Check sheet for the drawn part. Datum: minimum x, y, z corner. Units: mm. Round coordinates to 2 decimals unless told otherwise and drop trailing zeros. Loops run counter-clockwise (first coordinate to the right, second up) from the corner with the lowest first, then second, coordinate; pieces in that order, holes last. Notation, with made-up numbers: (64, 85) -> (121, 85) arc R19 ccw to (121, 109) -> close; hole circle Ø10 at (-18, -23.75). An arc over 180 degrees is marked (long way). Return JSON: item names as keys, results as strings.
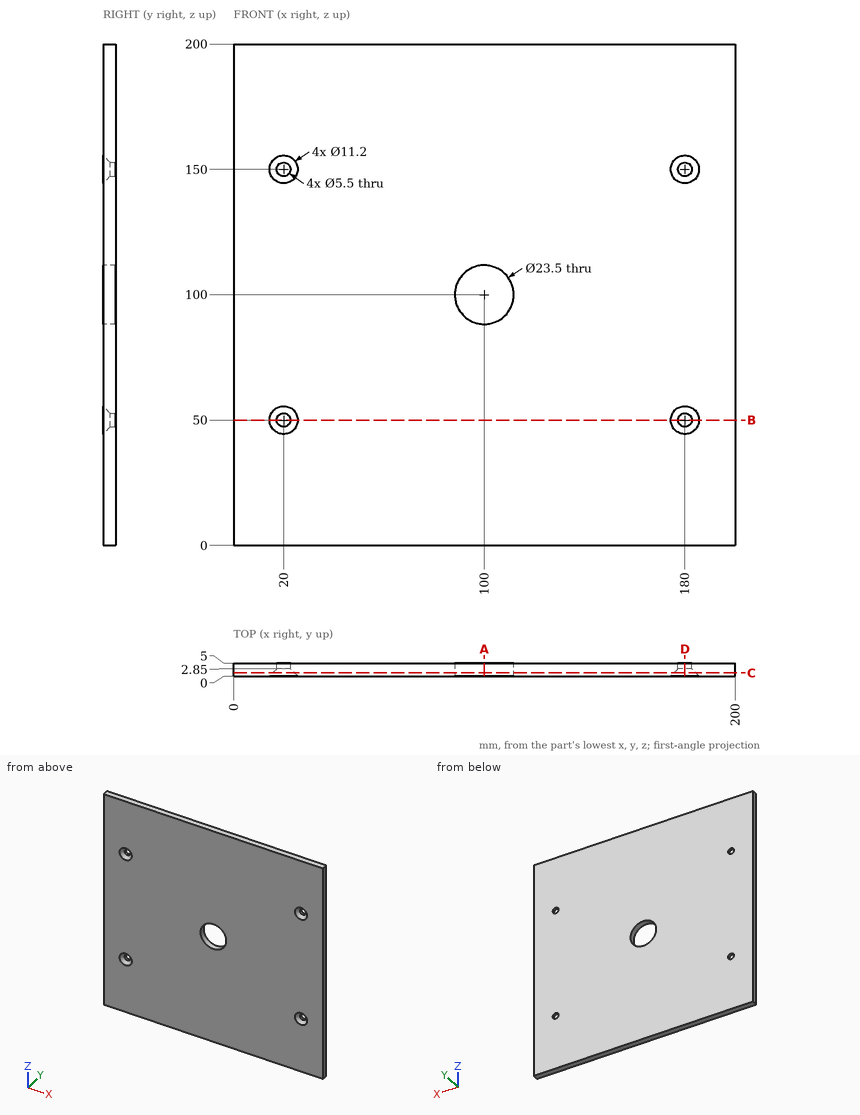
Q1. Go/stop test with flat-tipped pins: pin 1 (4.5 mm diameter, centred on x = 180, z = 150, fed in from +Y); pin 2 (10 mm diameter, centred on x = 163.5, z = 29, fed in from -Y). Record where each tip stops, or that it passes through.
Results list:
{"pin 1": "through", "pin 2": "y = 0"}
Q2. Section check A-A (x = 100). Record the boundary of the cut face in (y, z), then the cut area to 4 significant figures.
Results list:
{"outline": "(0, 0) -> (5, 0) -> (5, 88.25) -> (0, 88.25) -> close; (0, 111.75) -> (5, 111.75) -> (5, 200) -> (0, 200) -> close", "area": "882.5 mm^2"}
Q3. Material ranges on line 1 (Z direction, x = 179.5, y = 4.55); line 2 (X direction, y = 3.65, z = 150); line 3 (Z direction, x = 100, y = 1.4), recorded low to high.
Results list:
{"line 1": "0 to 47.3, 52.7 to 147.3, 152.7 to 200", "line 2": "0 to 17.25, 22.75 to 177.25, 182.75 to 200", "line 3": "0 to 88.25, 111.75 to 200"}
Q4. Section check D-D (x = 180). Record the boundary of the cut face in (y, z), then the cut area to 3 significant figures.
Results list:
{"outline": "(0, 0) -> (5, 0) -> (5, 47.25) -> (2.85, 47.25) -> (0, 44.4) -> close; (0, 55.6) -> (2.85, 52.75) -> (5, 52.75) -> (5, 147.25) -> (2.85, 147.25) -> (0, 144.4) -> close; (0, 155.6) -> (2.85, 152.75) -> (5, 152.75) -> (5, 200) -> (0, 200) -> close", "area": "929 mm^2"}
Q5. Section check C-C (y = 1.25). Record the boundary of the cut face in (x, z), then the cut area to 3 significant figures.
Results list:
{"outline": "(0, 0) -> (200, 0) -> (200, 200) -> (0, 200) -> close; hole circle Ø8.7 at (20, 50); hole circle Ø8.7 at (20, 150); hole circle Ø23.5 at (100, 100); hole circle Ø8.7 at (180, 50); hole circle Ø8.7 at (180, 150)", "area": "39,300 mm^2"}
Q6. Section check B-B (z = 50). Record the boundary of the cut face in (x, y), then the cut area to 3 significant figures.
Results list:
{"outline": "(0, 0) -> (14.4, 0) -> (17.25, 2.85) -> (17.25, 5) -> (0, 5) -> close; (22.75, 2.85) -> (25.6, 0) -> (174.4, 0) -> (177.25, 2.85) -> (177.25, 5) -> (22.75, 5) -> close; (182.75, 2.85) -> (185.6, 0) -> (200, 0) -> (200, 5) -> (182.75, 5) -> close", "area": "929 mm^2"}
